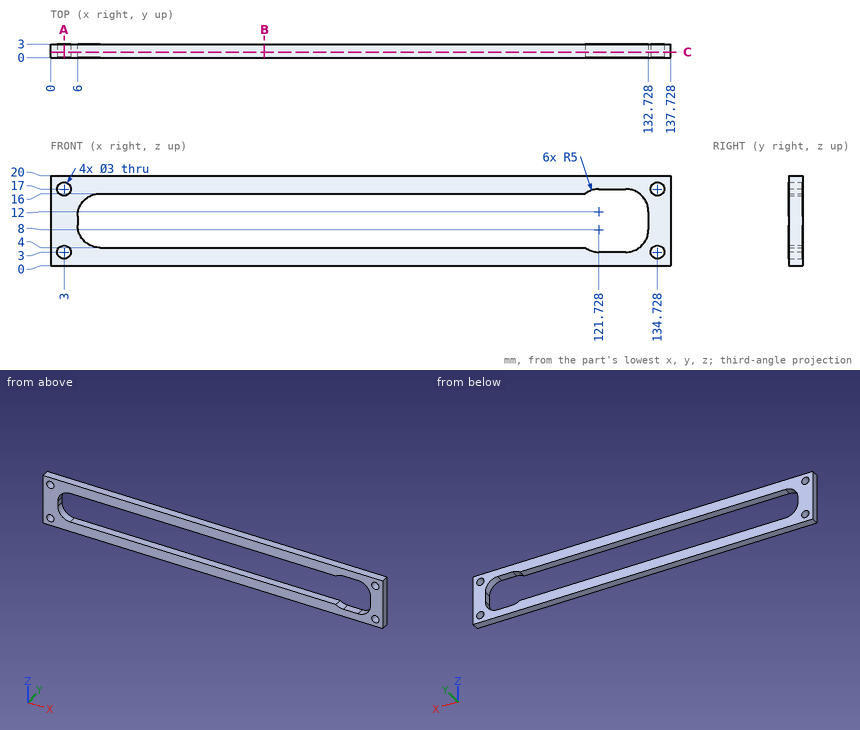
Geometry check sheet. Reference: drawing and pictorial views, mm from the part's lowest x, y, z. Round coordinates to 2 decimals unless told otherwise and drop trailing zeros. Write each loop counter-clockwise with the first axis right and the second up, starting at its lowest first coordinate (ties: lowest second). Pieces come first, ordered by that corner, then holes. Notation, with made-up numbers: (-10.75, 57) -> (-4.75, 57) arc R22 ccw to (-4.75, 84) -> close; hole circle Ø8 at (-31, -13.75). An arc over 180 degrees is marked (long way). Answer as CSV lines item,"result". Start each with the question number.
1) Section check A-A on x = 3. Enter the section's corners in (y, z), and give its area (3 significant figures).
2) Section check C-C on y = 1.2. Enter the section's corners in (x, z).
3) Go/stop test with a flat-tipped pin: P1, Ø2.5, axis at x = 3, z = 3, coming from the -Y side. Record where the tip stops, or that it passes through.
4) Section check B-B on x = 47.5. Enter the section's corners in (y, z), and give its area (3 significant figures).
5) Material ranges on line 1 (Z direction, x = 3, y = 1.25); line 2 (X direction, y = 2.6, z = 10.75); line 3 (Z direction, x = 97, y = 1.7), recorded low to high. Write a range as from..to.
Found:
1,outline,"(0, 0) -> (3, 0) -> (3, 1.5) -> (0, 1.5) -> close; (0, 4.5) -> (3, 4.5) -> (3, 15.5) -> (0, 15.5) -> close; (0, 18.5) -> (3, 18.5) -> (3, 20) -> (0, 20) -> close"
1,area,"42.0 mm^2"
2,outline,"(0, 0) -> (137.73, 0) -> (137.73, 20) -> (0, 20) -> close; hole circle Ø3 at (3, 3); hole circle Ø3 at (3, 17); hole (6, 9) arc R5 ccw to (11, 4) -> (118.73, 4) arc R5 ccw to (121.73, 3) -> (127.73, 3) arc R5 ccw to (132.73, 8) -> (132.73, 12) arc R5 ccw to (127.73, 17) -> (121.73, 17) arc R5 ccw to (118.73, 16) -> (11, 16) arc R5 ccw to (6, 11) -> close; hole circle Ø3 at (134.73, 3); hole circle Ø3 at (134.73, 17)"
3,P1,"passes through"
4,outline,"(0, 0) -> (3, 0) -> (3, 4) -> (0, 4) -> close; (0, 16) -> (3, 16) -> (3, 20) -> (0, 20) -> close"
4,area,"24.0 mm^2"
5,line 1,"z = 0..1.5, 4.5..15.5, 18.5..20"
5,line 2,"x = 0..6, 132.73..137.73"
5,line 3,"z = 0..4, 16..20"
